Source: CAD feature listing. Evaluate the final solid. Frame: model axes, mm. Round coordinates to 2 decimals unless told otherwise and drop trailing zeros. Order: outer loops, then holes, each group sorted by start corner. A loop starts at its lowest first (then second) coordinate and runs counter-clockwise, first axis right, second up. Notation, with made-up numbers: (-35, 55) -> (0, 55) arc R21 cw to (0, 63) -> close; hole circle Ø11 at (-23.5, 86.5). An arc over 180 degrees is marked (long way). Write item = value, one per line. Start each with the question number.
(1) Cut plane A-A on x = 10. Return the cut outline in (y, z), then the cut area to 3 significant figures.
(2) Cut plane D-D on z = 2.2. Give the number of separate pieces and of enclosed holes in the cut face, then the cut area to 3 significant figures.
(3) Ray query, line 1 (Y direction, x = -37.5, z = 1.25); line 2 (X direction, y = 12.5, z = 0.35); line 3 (X direction, y = 11.5, z = 0.2). Return the intervals inside material, ascending.
(4) Cut plane C-C on x = -37.5. Return the cut outline in (y, z), then the cut area to 3 significant figures.
(5) Cut plane B-B on y = 9.5. Return the cut outline in (x, z), then the cut area to 3 significant figures.
(6) Contact query for flat-ended pins moving along their axis: pin 1 Ø2 at (x, z) = (-33.5, 3) entering from -Y; pin 2 Ø5 at (x, y) = (20, 0) entering from +Z; pin 3 Ø1.2 at (x, z) = (17, 1.5) entering from +Y. Output: stop coordinate, or through.
from build123d import *

# Parameters (mm, degrees)
SKETCH_1_R               = 2.65
SKETCH_1_R_2             = 2.15
EXTRUDE_1_DEPTH          = 4
FILLET_1_R               = 5
CUT_EXTRUDE_1_DEPTH      = 73.782209365
FILLET_2_R               = 3
CUT_EXTRUDE_2_DEPTH      = 73.782209365
CUT_EXTRUDE_2_DEPTH_BACK = 73.782209365
FILLET_4_R               = 1.5
FILLET_6_R               = 3


with BuildPart() as part:
    # 草图1 → 凸台-拉伸1 (new body)
    with BuildSketch(Plane.XY):
        Polygon((-45, 17.5), (65, 17.5), (65, -22.5), (30, -22.5), (30, -32.5), (-10, -32.5), (-10, -22.5), (-45, -22.5), align=None)
        with Locations((20, 0)):
            Circle(SKETCH_1_R, mode=Mode.SUBTRACT)
        Circle(SKETCH_1_R, mode=Mode.SUBTRACT)
        with Locations((57.5, 13)):
            Circle(SKETCH_1_R_2, mode=Mode.SUBTRACT)
        with Locations((57.5, -12)):
            Circle(SKETCH_1_R_2, mode=Mode.SUBTRACT)
        with Locations(Location((-37.5, -12, 0), (0, 0, 180))):
            Circle(SKETCH_1_R_2, mode=Mode.SUBTRACT)
        with Locations(Location((-37.5, 13, 0), (0, 0, 180))):
            Circle(SKETCH_1_R_2, mode=Mode.SUBTRACT)
        with Locations((10, -27.5)):
            Circle(SKETCH_1_R, mode=Mode.SUBTRACT)
    extrude(amount=EXTRUDE_1_DEPTH)

    # 圆角1
    fillet_1_edges = [part.edges().sort_by_distance(p)[0] for p in [
        (30, -22.5, 2),
        (-45, 17.5, 2),
        (-45, -22.5, 2),
        (65, 17.5, 2),
        (65, -22.5, 2),
        (30, -32.5, 2),
        (-10, -32.5, 2),
        (-10, -22.5, 2),
    ]]
    fillet(fillet_1_edges, radius=FILLET_1_R - 0.0001)  # a hair under: the kernel refuses the full size

    # 草图3 → 切除-拉伸1 (cut, through all)
    with BuildSketch(Plane.XY.offset(4)):
        Polygon((-25, 17.5), (-15, 7.5), (35, 7.5), (45, 17.5), align=None)
    extrude(amount=-CUT_EXTRUDE_1_DEPTH, mode=Mode.SUBTRACT)

    # 圆角2
    fillet_2_edges = [part.edges().sort_by_distance(p)[0] for p in [
        (-25, 17.5, 2),
        (45, 17.5, 2),
        (35, 7.5, 2),
        (-15, 7.5, 2),
    ]]
    fillet(fillet_2_edges, radius=FILLET_2_R)

    # 草图4 → 切除-拉伸2 (cut, two sides: drawn at the far end of the back side and taken through both)
    with BuildSketch(Plane.XY.offset(4).offset(-CUT_EXTRUDE_2_DEPTH_BACK)):
        Polygon((38.743514733, 2.264213721), (23.108666515, -3.155866994), (14, -21.5), align=None)
        Polygon((27.981910241, -17.424640848), (53.5, -9.097685243), (53.5, 4.332888314), align=None)
        Polygon((-33.5, -9.097685243), (-33.5, 4.332888314), (-7.981910241, -17.424640848), align=None)
        Polygon((-18.743514733, 2.264213721), (-3.108666515, -3.155866994), (6, -21.5), align=None)
    extrude(amount=CUT_EXTRUDE_2_DEPTH + CUT_EXTRUDE_2_DEPTH_BACK, mode=Mode.SUBTRACT)

    # 圆角4
    fillet_4_edges = [part.edges().sort_by_distance(p)[0] for p in [
        (53.5, 4.332888314, 2),
        (53.5, -9.097685243, 2),
        (27.981910241, -17.424640848, 2),
        (-7.981910241, -17.424640848, 2),
        (-33.5, -9.097685243, 2),
        (-33.5, 4.332888314, 2),
        (38.743514733, 2.264213721, 2),
        (14, -21.5, 2),
        (-18.743514733, 2.264213721, 2),
        (6, -21.5, 2),
    ]]
    fillet(fillet_4_edges, radius=FILLET_4_R)

    # 圆角6
    fillet_6_edges = [part.edges().sort_by_distance(p)[0] for p in [
        (-3.108666515, -3.155866994, 2),
        (23.108666515, -3.155866994, 2),
    ]]
    fillet(fillet_6_edges, radius=FILLET_6_R)


solid = part.part
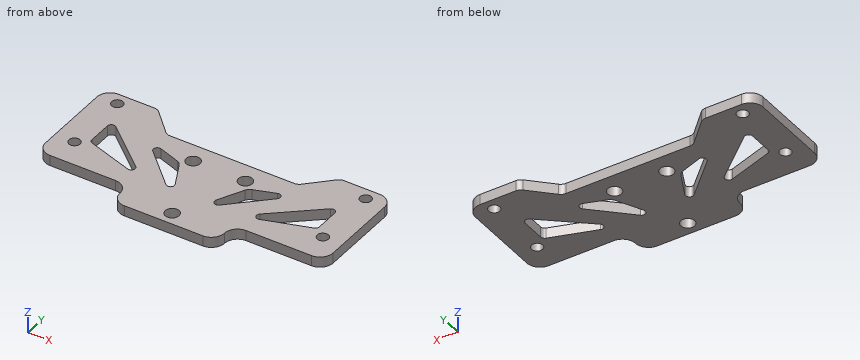
Evaluation:
q1.outline = (-32.5, 0) -> (-30.15, 0) -> (-30.15, 4) -> (-32.5, 4) -> close; (-24.85, 0) -> (7.5, 0) -> (7.5, 4) -> (-24.85, 4) -> close
q1.area = 139 mm^2
q2.separate_pieces = 1
q2.enclosed_holes = 11
q2.area = 3,530 mm^2
q3.line_1 = -22.5 to -14.15, -9.85 to 10.85, 15.15 to 17.5
q3.line_2 = -45 to -39.59, -35.41 to -20, 40 to 55.41, 59.59 to 65
q3.line_3 = -45 to -39.04, -35.96 to -19, 39 to 55.96, 59.04 to 65
q4.outline = (-22.5, 0) -> (-14.15, 0) -> (-14.15, 4) -> (-22.5, 4) -> close; (-9.85, 0) -> (10.85, 0) -> (10.85, 4) -> (-9.85, 4) -> close; (15.15, 0) -> (17.5, 0) -> (17.5, 4) -> (15.15, 4) -> close
q4.area = 126 mm^2
q5.outline = (-45, 0) -> (-17, 0) -> (-17, 4) -> (-45, 4) -> close; (37, 0) -> (65, 0) -> (65, 4) -> (37, 4) -> close
q5.area = 224 mm^2
q6.pin_1 = -22.5
q6.pin_2 = through
q6.pin_3 = 7.5
